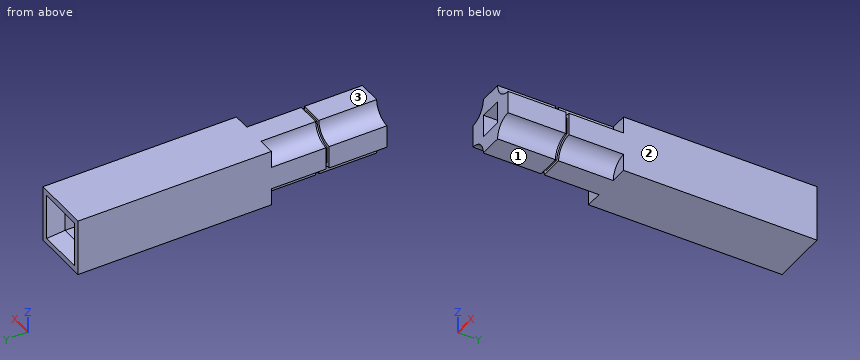
Autodesk Inventor part; units mm, degrees
ref_plane "YZ Plane" through (0, 0, 0) normal (1, 0, 0) x (0, 1, 0)
ref_plane "XZ Plane" through (0, 0, 0) normal (0, 1, 0) x (-1, 0, 0)
ref_plane "XY Plane" through (0, 0, 0) normal (0, 0, 1) x (1, 0, 0)
sketch "Sketch1" plane through (0, 0, 0) normal (0, 1, 0) x (-1, 0, 0)
  line L0 (1.27, 1.25) -> (-1.27, 1.25)
  line L1 (-1.27, 1.25) -> (-1.27, -1.25)
  line L2 (-1.27, -1.25) -> (1.27, -1.25)
  line L3 (1.27, -1.25) -> (1.27, 1.25)
  line L4 (1.27, 1.25) -> (-1.27, -1.25) construction
  line L5 (-1.27, 1.25) -> (1.27, -1.25) construction
  point P0 (0, 0)
  dimension "d0" = 2.54
  dimension "d1" = 2.5
extrude "Extrusion1" add sketch "Sketch1" along normal blind 8.5
sketch "Sketch2" plane through (0, 0, 0) normal (0, -1, 0) x (1, 0, 0)
  line L0 (-1.27, 1.25) -> (1.27, 1.25)
  arc A0 (0.52, 1.25) -> (1.27, 0.5) centre (1.27, 1.25) ccw
  line L1 (-1.27, -1.25) -> (-1.27, 1.25)
  arc A1 (-1.27, 0.5) -> (-0.52, 1.25) centre (-1.27, 1.25) ccw
  arc A2 (-0.52, -1.25) -> (-1.27, -0.5) centre (-1.27, -1.25) ccw
  line L2 (1.27, -1.25) -> (-1.27, -1.25)
  arc A3 (1.27, -0.5) -> (0.52, -1.25) centre (1.27, -1.25) ccw
  line L3 (1.27, 1.25) -> (1.27, -1.25)
  line L4 (-1.27, -1.25) -> (-1.27, 1.25)
  line L5 (1.27, -1.25) -> (-1.27, -1.25)
  point P0 (0, 0)
  dimension "d4" = 0.75
extrude "Extrusion2" add sketch "Sketch2" along normal blind 2.4 contours L0 A0 L3 A3 L2 A2 L1 A1
sketch "Sketch3" plane through (0, -2.4, 0) normal (0, -1, 0) x (1, 0, 0)
  line L0 (-1.125, 1.125) -> (1.125, 1.125)
  line L1 (1.125, 1.125) -> (1.125, -1.125)
  line L2 (1.125, -1.125) -> (-1.125, -1.125)
  line L3 (-1.125, -1.125) -> (-1.125, 1.125)
  line L4 (-1.125, 1.125) -> (1.125, -1.125) construction
  line L5 (1.125, 1.125) -> (-1.125, -1.125) construction
  arc A0 (-1.125, 0.3618) -> (-0.3787, 1.125) centre (-1.27, 1.25) ccw
  arc A1 (0.3787, 1.125) -> (1.125, 0.3618) centre (1.27, 1.25) ccw
  arc A2 (-0.3787, -1.125) -> (-1.125, -0.3618) centre (-1.27, -1.25) ccw
  arc A3 (1.125, -0.3618) -> (0.3787, -1.125) centre (1.27, -1.25) ccw
  point P0 (0, 0)
  dimension "d7" = 2.25
  dimension "d8" = 0.9
  dimension "d9" = 0.9
  dimension "d10" = 0.9
  dimension "d11" = 0.9
extrude "Extrusion3" add sketch "Sketch3" along normal blind 0.14 contours L0 A1 L1 A3 L2 A2 L3 A0
sketch "Sketch4" plane through (0, -2.54, 0) normal (0, -1, 0) x (1, 0, 0)
  line L0 (0.52, 1.25) -> (-0.52, 1.25)
  arc A0 (-1.27, 0.5) -> (-0.52, 1.25) centre (-1.27, 1.25) ccw
  line L1 (-1.27, 0.5) -> (-1.27, -0.5)
  arc A1 (-0.52, -1.25) -> (-1.27, -0.5) centre (-1.27, -1.25) ccw
  line L2 (-0.52, -1.25) -> (0.52, -1.25)
  arc A2 (1.27, -0.5) -> (0.52, -1.25) centre (1.27, -1.25) ccw
  line L3 (1.27, -0.5) -> (1.27, 0.5)
  arc A3 (0.52, 1.25) -> (1.27, 0.5) centre (1.27, 1.25) ccw
  point P0 (0, 0)
extrude "Extrusion4" add sketch "Sketch4" along normal blind 2.54
sketch "Sketch5" plane through (0, 8.5, 0) normal (0, 1, 0) x (1, 0, 0)
  line L0 (-0.5, 0.5) -> (0.5, 0.5)
  line L1 (0.5, 0.5) -> (0.5, -0.5)
  line L2 (0.5, -0.5) -> (-0.5, -0.5)
  line L3 (-0.5, -0.5) -> (-0.5, 0.5)
  line L4 (-0.5, 0.5) -> (0.5, -0.5) construction
  line L5 (0.5, 0.5) -> (-0.5, -0.5) construction
  point P0 (0, 0)
  dimension "d16" = 1
extrude "Extrusion5" cut sketch "Sketch5" against normal through all
chamfer "Chamfer1" distance 0.5 angle 45 4 edges at (0, 8.5, -0.5) (-0.5, 8.5, 0) (0, 8.5, 0.5) (0.5, 8.5, 0)
properties part number "SMT GPIO Female Header 2x20"
Design review of the part built by this model. Coordinates are the model's own, in mm. Face numbers are marked on the shaded views. Coordinates: 2 decimals unless noted, no trailing zeros. Order: outer loops, then holes, each group sorted by start corner. A loop starts at its lowest first (then second) coordinate and runs counter-clockwise, first axis right, second up. Notation, with made-up numbers: (14, -33) -> (24, -33) arc R26 cw to (24, -15) -> close; hole circle Ø10 at (0, 85). An arc over 180 degrees is marked (long way). Use one line per item in the form item = value. Start each with the question number.
(1) Add section C-C on x = 0.2. State the section outline as (y, z) points (3 decimals).
(2) For probe 1 along Z at (x, y) = (0, 3.75); probe 2 along X at (y, z) = (6.5, 0); probe 3 along Y at (x, z) = (1, -1.05), list the stretches that pass through material, from the lowest coordinate up.
(3) The part is to be moulded in two halves that separate along Z. For the marked faces 1, 2 and 3, say which applies: +Z half, -Z half, draft (parallel to the pull), parting line (faces both ways), or undercut.
(4) Add section A-A on z = 0.2. State the section outline as (x, y) points (3 decimals), plus the area to 3 significant figures.
(5) Add section B-B on y = -4. State the section outline as (x, z) points, plus the area to 3 significant figures.
(6) Add section D-D on x = -0.75. State the section outline as (y, z) points, plus the area to 3 significant figures.
Answer block:
q1.outline = (-5.08, -1.25) -> (-2.54, -1.25) -> (-2.54, -1.125) -> (-2.4, -1.125) -> (-2.4, -1.25) -> (8.5, -1.25) -> (8.5, -1) -> (8, -0.5) -> (-5.08, -0.5) -> close; (-5.08, 0.5) -> (8, 0.5) -> (8.5, 1) -> (8.5, 1.25) -> (-2.4, 1.25) -> (-2.4, 1.125) -> (-2.54, 1.125) -> (-2.54, 1.25) -> (-5.08, 1.25) -> close
q2.probe_1 = -1.25 to -0.5, 0.5 to 1.25
q2.probe_2 = -1.27 to -0.5, 0.5 to 1.27
q2.probe_3 = 0 to 8.5
q3.face_1 = -Z half
q3.face_2 = draft
q3.face_3 = +Z half
q4.outline = (-1.27, -5.08) -> (-0.5, -5.08) -> (-0.5, 8) -> (-1, 8.5) -> (-1.27, 8.5) -> (-1.27, -2.4) -> (-1.125, -2.4) -> (-1.125, -2.54) -> (-1.27, -2.54) -> close; (0.5, -5.08) -> (1.27, -5.08) -> (1.27, -2.54) -> (1.125, -2.54) -> (1.125, -2.4) -> (1.27, -2.4) -> (1.27, 8.5) -> (1, 8.5) -> (0.5, 8) -> close
q4.area = 20.6 mm²
q5.outline = (-1.27, -0.5) arc R0.75 cw to (-0.52, -1.25) -> (0.52, -1.25) arc R0.75 cw to (1.27, -0.5) -> (1.27, 0.5) arc R0.75 cw to (0.52, 1.25) -> (-0.52, 1.25) arc R0.75 cw to (-1.27, 0.5) -> close; hole (-0.5, -0.5) -> (0.5, -0.5) -> (0.5, 0.5) -> (-0.5, 0.5) -> close
q5.area = 3.58 mm²
q6.outline = (-5.08, -0.71) -> (-2.54, -0.71) -> (-2.54, -0.52) -> (-2.4, -0.52) -> (-2.4, -0.71) -> (0, -0.71) -> (0, -1.25) -> (8.5, -1.25) -> (8.5, -1) -> (8.25, -0.75) -> (8.25, 0.75) -> (8.5, 1) -> (8.5, 1.25) -> (0, 1.25) -> (0, 0.71) -> (-2.4, 0.71) -> (-2.4, 0.52) -> (-2.54, 0.52) -> (-2.54, 0.71) -> (-5.08, 0.71) -> close
q6.area = 28.0 mm²
